For this review, use the dimensioned drawing (mm, ordinates from the lowest corner) and the shaded views. Round coordinates to 2 decimals unless told otherwise and drop trailing zeros. Order: outer loops, then holes, each group sorted by start corner. A loop starts at its lowest first (then second) coordinate and runs counter-clockwise, first axis right, second up. Notation, with made-up numbers: (31.5, 82) - (47.5, 82) arc R26 cw to (47.5, 96) - close; hole circle Ø9 at (-31.75, -27.75). An arc over 180 degrees is marked (long way). Write item = value, one per line.
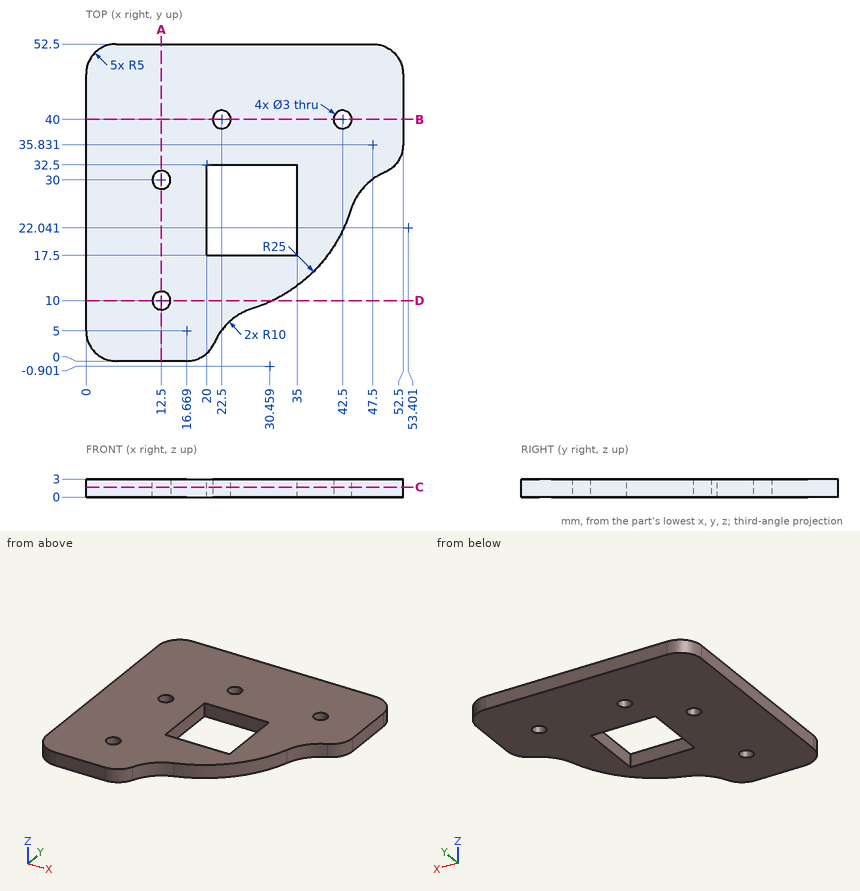
Item 1: Take a section at D-D, the plane y = 10. State the section outline as (x, z) points.
Data:
outline = (0, 0) - (11, 0) - (11, 3) - (0, 3) - close; (14, 0) - (30.9, 0) - (30.9, 3) - (14, 3) - close
Item 2: Take a section at A-A, the plane x = 12.5. State the section outline as (y, z) points.
Data:
outline = (0, 0) - (8.5, 0) - (8.5, 3) - (0, 3) - close; (11.5, 0) - (28.5, 0) - (28.5, 3) - (11.5, 3) - close; (31.5, 0) - (52.5, 0) - (52.5, 3) - (31.5, 3) - close
Item 3: For line 1 along Y through (x, z) = (12.5, 2.05); line 2 along Y through (x, z) = (22.5, 2.15) (1 decimal); line 3 along X through (y, z) = (10, 2.8) (1 decimal), list the stretches that pass through material, from the lowest coordinate up. Write a range as [from, to].
Data:
line_1 = [0, 8.5], [11.5, 28.5], [31.5, 52.5]
line_2 = [5.2, 17.5], [32.5, 38.5], [41.5, 52.5]
line_3 = [0, 11], [14, 30.9]
Item 4: Take a section at C-C, the plane z = 1.65. State the section outline as (x, y) points (1 decimal).
Data:
outline = (0, 5) arc R5 ccw to (5, 0) - (16.7, 0) arc R5 ccw to (21.3, 3) arc R10 cw to (27.5, 8.6) arc R25 ccw to (43.9, 25) arc R10 cw to (49.5, 31.2) arc R5 ccw to (52.5, 35.8) - (52.5, 47.5) arc R5 ccw to (47.5, 52.5) - (5, 52.5) arc R5 ccw to (0, 47.5) - close; hole circle Ø3 at (12.5, 10); hole circle Ø3 at (12.5, 30); hole (20, 17.5) - (35, 17.5) - (35, 32.5) - (20, 32.5) - close; hole circle Ø3 at (22.5, 40); hole circle Ø3 at (42.5, 40)
Item 5: Take a section at B-B, the plane y = 40. State the section outline as (x, z) points.
Data:
outline = (0, 0) - (21, 0) - (21, 3) - (0, 3) - close; (24, 0) - (41, 0) - (41, 3) - (24, 3) - close; (44, 0) - (52.5, 0) - (52.5, 3) - (44, 3) - close
Item 6: Insertion check: P1, Ø1.8, axis at x = 42.5, y = 40, coming from the -Z side; P2, Ø0.9, axis at y = 28, z = 2, coming from the +X side (1 decimal). Each pin has a flat end and moves straight along its axis. Give the tip position at first contact, or say it passes through.
Data:
P1 = through
P2 = 45.7
